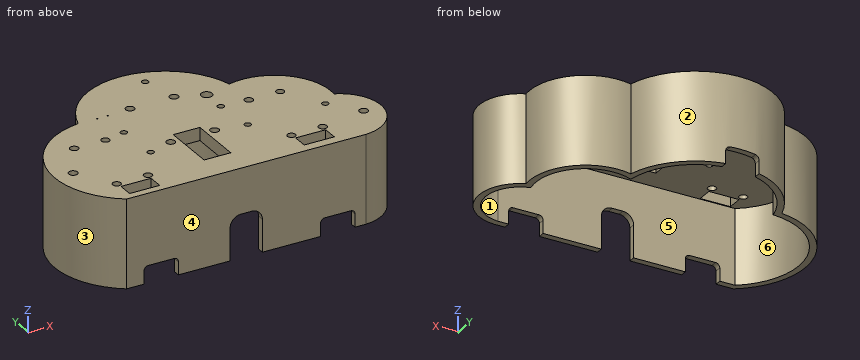
```python
from build123d import *

# Parameters (mm, degrees)
BOSS_EXTRU_1_DEPTH           = 6
BOSS_EXTRU_2_DEPTH           = 6
BOSS_EXTRU_2_DEPTH_BACK      = 35
ENL_V_MAT_EXTRU_2_REACH      = 128.442
ESQUISSE5_W                  = 15
ESQUISSE5_H                  = 20
CONG_1_R                     = 5
ENL_V_MAT_EXTRU_3_REACH      = 128.442
ESQUISSE6_W                  = 16
ESQUISSE6_H                  = 8
ENL_V_MAT_EXTRU_4_REACH      = 105.054
ENL_V_MAT_EXTRU_4_END_RADIUS = 36
ESQUISSE7_W                  = 16
ESQUISSE7_H                  = 8
CONG_2_R                     = 2
ESQUISSE10_R                 = 2
ESQUISSE10_R_2               = 1.5
ESQUISSE10_R_3               = 1.863501178
ESQUISSE10_R_4               = 1.93430269
ESQUISSE10_R_5               = 1.939737899
ESQUISSE10_R_6               = 1.854627201
ESQUISSE10_R_7               = 2.55
ESQUISSE10_W                 = 12.4
ESQUISSE10_H                 = 25
ESQUISSE10_W_2               = 0.5
ESQUISSE10_H_2               = 0.5
ENL_V_MAT_EXTRU_6_DEPTH      = 104.053910907


with BuildPart() as part:
    # Esquisse2 → Boss.-Extru.1 (new body)
    with BuildSketch(Plane.XY):
        with BuildLine():
            Line((-48.608879521, -52.647186827), (61.474409074, -52.647186827))
            ThreePointArc((61.474409074, -52.647186827), (76.298877159, -38.117787006), (64.302141331, -21.178287526))
            ThreePointArc((64.302141331, -21.178287526), (56.703051449, 1.556908822), (33.007522473, 5.184197975))
            ThreePointArc((33.007522473, 5.184197975), (1.426097383, 33.335688366), (-31.902467285, 7.276148862))
            ThreePointArc((-31.902467285, 7.276148862), (-61.424642208, -16.783685992), (-48.608879521, -52.647186827))
        make_face()
    extrude(amount=BOSS_EXTRU_1_DEPTH)

    # Esquisse3 → Boss.-Extru.2 (add, two sides: drawn at the far end of the back side and taken through both)
    with BuildSketch(Plane.XY.offset(-BOSS_EXTRU_2_DEPTH_BACK)):
        with BuildLine():
            Line((-49.534861191, -55.647186827), (61.574237986, -55.647186827))
            ThreePointArc((61.574237986, -55.647186827), (79.101164774, -39.829765432), (67.696496182, -19.158105688))
            ThreePointArc((67.696496182, -19.158105688), (58.974577176, 3.560965394), (35.280810603, 9.113756361))
            ThreePointArc((35.280810603, 9.113756361), (0.847370614, 36.349555954), (-34.306277728, 10.0499062))
            ThreePointArc((-34.306277728, 10.0499062), (-64.707061967, -17.516732287), (-49.534861191, -55.647186827))
        make_face()
        with BuildLine():
            Line((-48.608879521, -52.647186827), (61.474409074, -52.647186827))
            ThreePointArc((61.474409074, -52.647186827), (76.298877159, -38.117787006), (64.302141331, -21.178287526))
            ThreePointArc((64.302141331, -21.178287526), (56.703051449, 1.556908822), (33.007522473, 5.184197975))
            ThreePointArc((33.007522473, 5.184197975), (1.426097383, 33.335688366), (-31.902467285, 7.276148862))
            ThreePointArc((-31.902467285, 7.276148862), (-61.424642208, -16.783685992), (-48.608879521, -52.647186827))
        make_face(mode=Mode.SUBTRACT)
    extrude(amount=BOSS_EXTRU_2_DEPTH + BOSS_EXTRU_2_DEPTH_BACK)

    # Esquisse5 → Enlèv. mat.-Extru.2 (cut, up to next)
    with BuildSketch(Plane.XZ.offset(55.647186827), mode=Mode.PRIVATE) as enl_v_mat_extru_2_sk1:
        with Locations((6.019688397, -25)):
            Rectangle(ESQUISSE5_W, ESQUISSE5_H)
    enl_v_mat_extru_2_tool1 = extrude(enl_v_mat_extru_2_sk1.sketch, amount=-ENL_V_MAT_EXTRU_2_REACH, mode=Mode.PRIVATE) & part.part
    add(enl_v_mat_extru_2_tool1.solids().sort_by_distance((6.019688, -55.647187, -25))[0], mode=Mode.SUBTRACT)

    # Congé1
    cong_1_edges = [part.edges().sort_by_distance(p)[0] for p in [
        (13.519688397, -54.147186827, -15),
        (-1.480311603, -54.147186827, -15),
    ]]
    fillet(cong_1_edges, radius=CONG_1_R)

    # Esquisse6 → Enlèv. mat.-Extru.3 (cut, up to next)
    with BuildSketch(Plane.XZ.offset(55.647186827), mode=Mode.PRIVATE) as enl_v_mat_extru_3_sk1:
        with Locations((-33.480311603, -31)):
            Rectangle(ESQUISSE6_W, ESQUISSE6_H)
    enl_v_mat_extru_3_tool1 = extrude(enl_v_mat_extru_3_sk1.sketch, amount=-ENL_V_MAT_EXTRU_3_REACH, mode=Mode.PRIVATE) & part.part
    # Esquisse6 → Enlèv. mat.-Extru.3 (cut, up to next)
    with BuildSketch(Plane.XZ.offset(55.647186827), mode=Mode.PRIVATE) as enl_v_mat_extru_3_sk2:
        with Locations((48.519688397, -31)):
            Rectangle(ESQUISSE6_W, ESQUISSE6_H)
    enl_v_mat_extru_3_tool2 = extrude(enl_v_mat_extru_3_sk2.sketch, amount=-ENL_V_MAT_EXTRU_3_REACH, mode=Mode.PRIVATE) & part.part
    add(enl_v_mat_extru_3_tool1.solids().sort_by_distance((-33.480312, -55.647187, -31))[0], mode=Mode.SUBTRACT)
    add(enl_v_mat_extru_3_tool2.solids().sort_by_distance((48.519688, -55.647187, -31))[0], mode=Mode.SUBTRACT)

    # Enlèv. mat.-Extru.4: up to this cylinder (the profile starts inside it)
    enl_v_mat_extru_4_end = Plane(origin=(0.363109154, 0.352813173, -31), z_dir=(0, 0, -1)) * Cylinder(ENL_V_MAT_EXTRU_4_END_RADIUS, 283.108, mode=Mode.PRIVATE)
    # Esquisse7 → Enlèv. mat.-Extru.4 (cut, up to the surface)
    with BuildSketch(Plane(origin=(0, 0, 0), x_dir=(1, 0, 0), z_dir=(0, 1, 0)), mode=Mode.PRIVATE) as enl_v_mat_extru_4_sk1:
        with Locations((-1.480311603, 31)):
            Rectangle(ESQUISSE7_W, ESQUISSE7_H)
    enl_v_mat_extru_4_tool1 = extrude(enl_v_mat_extru_4_sk1.sketch, amount=ENL_V_MAT_EXTRU_4_REACH, mode=Mode.PRIVATE) & enl_v_mat_extru_4_end
    add(enl_v_mat_extru_4_tool1.solids().sort_by_distance((-1.480312, 0, -31))[0], mode=Mode.SUBTRACT)

    # Congé2
    cong_2_edges = [part.edges().sort_by_distance(p)[0] for p in [
        (-9.480311603, 33.415741443, -27),
        (6.519688397, 34.297950888, -27),
        (40.519688397, -54.147186827, -27),
        (56.519688397, -54.147186827, -27),
        (-41.480311603, -54.147186827, -27),
        (-25.480311603, -54.147186827, -27),
    ]]
    fillet(cong_2_edges, radius=CONG_2_R)

    # Esquisse10 → Enlèv. mat.-Extru.6 (cut, through all)
    with BuildSketch(Plane.XY):
        with Locations((-57.135320842, -25.647186827)):
            Circle(ESQUISSE10_R)
        with Locations((10.563109154, -22.147186827)):
            Circle(ESQUISSE10_R)
        with Locations((10.563109154, 10.752813173)):
            Circle(ESQUISSE10_R)
        with Locations((-9.836890846, 10.752813173)):
            Circle(ESQUISSE10_R)
        with Locations((-22.136890846, -5.697186827)):
            Circle(ESQUISSE10_R_2)
        with Locations((22.863109154, -5.697186827)):
            Circle(ESQUISSE10_R_2)
        with Locations((-9.836890846, -22.147186827)):
            Circle(ESQUISSE10_R)
        with Locations((70.864679158, -37.647186827)):
            Circle(ESQUISSE10_R)
        with Locations((6.864679158, 27.587526086)):
            Circle(ESQUISSE10_R_2)
        with Locations((-46.489752539, -42.38368966)):
            Circle(ESQUISSE10_R_3)
        with Locations((-31.89810954, -42.24093029)):
            Circle(ESQUISSE10_R_4)
        with Locations((-46.278226209, -7.591233185)):
            Circle(ESQUISSE10_R_5)
        with Locations((-31.810577097, -7.638641543)):
            Circle(ESQUISSE10_R_6)
        with Locations((-21.135320842, -25.647186827)):
            Circle(ESQUISSE10_R_2)
        with Locations((60.519688397, -24.647186827)):
            Circle(ESQUISSE10_R_2)
        with Locations((24.519688397, -24.647186827)):
            Circle(ESQUISSE10_R_2)
        with Locations((35.37678303, -6.591233185)):
            Circle(ESQUISSE10_R_5)
        with Locations((49.844432143, -6.638641543)):
            Circle(ESQUISSE10_R_6)
        with Locations((49.7568997, -41.24093029)):
            Circle(ESQUISSE10_R_4)
        with Locations((35.165256701, -41.38368966)):
            Circle(ESQUISSE10_R_3)
        with Locations((22.863109154, 5.752813173)):
            Circle(ESQUISSE10_R_7)
        with Locations((0.363109154, -29.697186827)):
            Rectangle(ESQUISSE10_W, ESQUISSE10_H)
        Polygon((-46.135320842, -49.647186827), (-46.135320842, -45.147186827), (-32.135320842, -45.147186827), (-32.135320842, -49.647186827), (-32.135320842, -52.147186827), (-46.135320842, -52.147186827), align=None)
        Polygon((35.519688397, -48.647186827), (35.519688397, -44.147186827), (49.519688397, -44.147186827), (49.519688397, -48.647186827), (49.519688397, -51.147186827), (35.519688397, -51.147186827), align=None)
        with Locations((-20.636890846, 9.852813173)):
            Rectangle(ESQUISSE10_W_2, ESQUISSE10_H_2)
        with Locations((-25.636890846, 9.852813173)):
            Rectangle(ESQUISSE10_W_2, ESQUISSE10_H_2)
    extrude(amount=ENL_V_MAT_EXTRU_6_DEPTH, mode=Mode.SUBTRACT)


solid = part.part
```
Here's how the part is built. I have some questions about the finished solid (model axes, mm). Face numbers are marked on the shaded views. A direction names the side the tool comes from. Round coordinates to 2 decimals unless told otherwise and drop trailing zeros. Write each loop counter-clockwise with the first axis right and the second up, starting at its lowest first coordinate (ties: lowest second). Pieces come first, ordered by that corner, then holes. Notation, with made-up numbers: M 33.5,88 L 54.5,88 A26 ccw 54.5,109 Z; hole C -2.5,0 d8. An arc over 180 degrees is marked long. Answer as CSV lines item,"result". Start each with the question number.
1. Suppose I cut it at C-C on x = -51.5. Write out the boundary of the cut face in (y, z).
2. Suppose I cut it at A-A on x = 11. Write out the boundary of the cut face in (y, z).
3. Suppose I cut it at D-D on z = -25.5. Write out the boundary of the cut face in (x, y).
4. I'm going to push flat-ended pins straight in: pin 1 Ø5 at (x, y) = (49.76, -41.24) entering from -Z; pin 2 Ø6 at (x, z) = (-23, 1.5) entering from +Y; pin 3 Ø2.5 at (x, y) = (10.56, 10.75) entering from -Z; pin 4 Ø6 at (x, z) = (-29, -26.5) entering from +Y. Where does each tip first touch, or does it pass through?
5. Thinking about a two-plate mould opening in X: for the marked faces 3, 4, 5 and 6, which applies, released by +X, released by -X, zero draft, split by the parting line, or undercut?
6. I need wall thicknesses on probe 1 along X at (y, z) = (-5, 0.5); probe 2 along Z at (x, y) = (41, -24.5); probe 3 along Y at (x, z) = (70.5, -15.5). Which ranges of each line are inside material? Lowest first, please.
7. On a 3-axis mill with a long thin cutter (end or side, diameter ignored), from which of +Z, -Z, +X, -X, +Y, -Y can I reach the whole of each face in a straight line? I mean the marked faces 1 and 2. Say none if no direction works.
8. Suppose I cut it at B-B on z = -10. Write out the boundary of the cut face in (x, y).
Check result:
1,outline,"M -54.25,-35 L -50.36,-35 L -50.36,0 L -0.93,0 L -0.93,-35 L 2.95,-35 L 2.95,6 L -54.25,6 Z"
2,outline,"M -55.65,-15.66 L -52.65,-15.66 L -52.65,0 L -24.1,0 L -24.1,6 L -55.65,6 Z; M -20.2,0 L 8.8,0 L 8.8,6 L -20.2,6 Z; M 12.7,0 L 31.59,0 L 31.59,-35 L 34.75,-35 L 34.75,6 L 12.7,6 Z"
3,outline,"M -49.53,-55.65 L -1.48,-55.65 L -1.48,-52.65 L -48.61,-52.65 A33 cw -31.9,7.28 A33 cw 33.01,5.18 A23 cw 64.3,-21.18 A16 cw 61.47,-52.65 L 13.52,-52.65 L 13.52,-55.65 L 61.57,-55.65 A19 ccw 67.7,-19.16 A26 ccw 35.28,9.11 A36 ccw -34.31,10.05 A36 ccw Z"
4,pin 1,"stops at z = 0"
4,pin 2,"stops at y = 30.04"
4,pin 3,"passes through"
4,pin 4,"stops at y = 24.87"
5,face 3,"released by -X"
5,face 4,"zero draft"
5,face 5,"undercut"
5,face 6,"undercut"
6,probe 1,"x = -59.13 to -23.47, -20.81 to 21.53, 24.19 to 34.27, 36.49 to 48.98, 50.71 to 65.43"
6,probe 2,"z = 0 to 6"
6,probe 3,"y = -52.76 to -49.06, -24.31 to -20.62"
7,face 1,"-Z"
7,face 2,"+Z, -Z, +Y"
8,outline,"M -49.53,-55.65 L 61.57,-55.65 A19 ccw 67.7,-19.16 A26 ccw 35.28,9.11 A36 ccw -34.31,10.05 A36 ccw Z; hole M -48.61,-52.65 L 61.47,-52.65 A16 ccw 64.3,-21.18 A23 ccw 33.01,5.18 A33 ccw -31.9,7.28 A33 ccw Z"
